Design review of the part built by this model. Coordinates are the model's own, in mm. A direction names the side the tool comes from. Give positions to 0.01 mm unless a question says otherwise; leave off trailing zeros. Loops run counter-clockwise (first coordinate to the right, second up) from the corner with the lowest first, then second, coordinate; pieces in that order, holes last. Notation, with made-up numbers: M 16.25,-18.5 L 21.25,-18.5 A18 cw 21.25,-3.5 Z; hole C 31.25,-38 d5. An arc over 180 degrees is marked long. Use CSV: the item, a comma, the result in double quotes.
from build123d import *

# Parameters (mm, degrees)
EXTRUDE_1_DEPTH     = 105
SKETCH_2_W          = 4
SKETCH_2_H          = 105
EXTRUDE_2_DEPTH     = 3
SKETCH_4_W          = 60
SKETCH_4_H          = 11
EXTRUDE_3_DEPTH     = 5
SKETCH_6_W          = 60
SKETCH_6_H          = 110
SKETCH_6_H_2        = 20
EXTRUDE_4_DEPTH     = 10
CUT_EXTRUDE_1_DEPTH = 4
SKETCH_9_R          = 2.25
CUT_EXTRUDE_2_DEPTH = 139.430487971


with BuildPart() as part:
    # 스케치1 → 보스-돌출1 (new body)
    with BuildSketch(Plane.XY):
        Polygon((-3, 0), (0, 0), (0, 4), (54, 4), (54, 0), (57, 0), (57, 8), (-3, 8), align=None)
    extrude(amount=EXTRUDE_1_DEPTH)

    # 스케치2 → 보스-돌출2 (add)
    with BuildSketch(Plane.XZ):
        with Locations((-1, 52.5)):
            Rectangle(SKETCH_2_W, SKETCH_2_H)
        with Locations((55, 52.5)):
            Rectangle(SKETCH_2_W, SKETCH_2_H)
    extrude(amount=EXTRUDE_2_DEPTH)

    # 스케치4 → 보스-돌출3 (add)
    with BuildSketch(Plane(origin=(0, 0, 0), x_dir=(-1, 0, 0), z_dir=(0, 0, -1))):
        with Locations((-27, 2.5)):
            Rectangle(SKETCH_4_W, SKETCH_4_H)
    extrude(amount=EXTRUDE_3_DEPTH)

    # 스케치6 → 보스-돌출4 (add)
    with BuildSketch(Plane(origin=(0, 8, 0), x_dir=(1, 0, 0), z_dir=(0, 1, 0))):
        with Locations((27, -50)):
            Rectangle(SKETCH_6_W, SKETCH_6_H)
        with Locations((27, -115)):
            Rectangle(SKETCH_6_W, SKETCH_6_H_2)
    extrude(amount=EXTRUDE_4_DEPTH)

    # 스케치8 → 컷-돌출1 (cut)
    with BuildSketch(Plane(origin=(0, 18, 0), x_dir=(1, 0, 0), z_dir=(0, 1, 0))):
        Polygon((23, -115.190598923), (23, -119.809401077), (27, -122.118802154), (31, -119.809401077), (31, -115.190598923), (27, -112.881197846), align=None)
    extrude(amount=-CUT_EXTRUDE_1_DEPTH, mode=Mode.SUBTRACT)

    # 스케치9 → 컷-돌출2 (cut, through all)
    with BuildSketch(Plane(origin=(0, 14, 0), x_dir=(1, 0, 0), z_dir=(0, 1, 0))):
        with Locations(Location((27, -117.5, 0), (0, 0, 270))):
            Circle(SKETCH_9_R)
    extrude(amount=-CUT_EXTRUDE_2_DEPTH, mode=Mode.SUBTRACT)


solid = part.part
(1) Clearance check with flat-ended pins moving along their axes: P1, Ø5, axis at x = 45, z = 109, coming from the -Y side; P2, Ø1.5, axis at x = 46, z = 36, coming from the -Y side; P3, Ø3, axis at x = 48, y = 0.5, coming from the +Z side. State where each tip first meets the part, or that it passes through.
A:
P1,"y = 8"
P2,"y = 4"
P3,"z = 0"
(2) Wall thickness on line 1 along X through (y, z) = (9.6, 117.5); line 2 along Z through (x, y) = (3.5, 1.25); line 3 along Y through (x, z) = (24, 39.5): over which ranges is each line inside the solid? List them lowest first. Write a range as [from, to].
A:
line 1,"[-3, 24.75], [29.25, 57]"
line 2,"[-5, 0]"
line 3,"[4, 18]"
(3) The part is to be moulded in two halves that separate along Z. For faces 5 (the flat face through (27, 13, 125)), 6 (the flat face through (1, -1, 52)), 7 (the flat face through (28, 14, 115)), say which applies: released by +Z, released by -Z, zero draft, split by the parting line, or undercut.
A:
face 5,"released by +Z"
face 6,"zero draft"
face 7,"undercut"
(4) We need section C-C on z = 9.5. State the section outline as (x, y) points.
A:
outline,"M -3,-3 L 1,-3 L 1,0 L 0,0 L 0,4 L 54,4 L 54,0 L 53,0 L 53,-3 L 57,-3 L 57,18 L -3,18 Z"
(5) Machinability: for faces 1 (the flat face through (53, -1, 52)), 2 (the flat face through (31, 16, 118)), 3 (the flat face through (27, 8, 115)), 4 (the flat face through (54, 2, 52)), which of the approach directions +Z, -Z, +X, -X, +Y, -Y give a long, thin tool a straight path to every point of the face, cutting with its end or side? Answer none if there is none.
A:
face 1,"+Z, -Y"
face 2,"+Y"
face 3,"+Z, +X, -X, -Y"
face 4,"+Z"
(6) We need section B-B on x = 9.5. State the section outline as (y, z) points, then the cut area to 4 significant figures.
A:
outline,"M -3,-5 L 18,-5 L 18,125 L 8,125 L 8,105 L 4,105 L 4,0 L -3,0 Z"
area,"1,775 mm²"
(7) We need section A-A on z = 117.5. State the section outline as (x, y) points, then the cut area to 3 significant figures.
A:
outline,"M -3,8 L 24.75,8 L 24.75,14 L 23,14 L 23,18 L -3,18 Z; M 29.25,8 L 57,8 L 57,18 L 31,18 L 31,14 L 29.25,14 Z"
area,"541 mm²"
